Could you check a few things on this model? Use its own coordinates, in mm. Face numbers are marked on the shaded views. A direction names the side the tool comes from. Give positions to 0.01 mm unless a question says otherwise; leave off trailing zeros. Order: outer loops, then holes, each group sorted by start corner. A loop starts at its lowest first (then second) coordinate and runs counter-clockwise, first axis right, second up. Notation, with made-up numbers: (51.5, -27) -> (107.5, -27) arc R28 ccw to (107.5, 1) -> close; hole circle Ø11 at (52, 26.5). An arc over 180 degrees is marked (long way). Write each question's results on one line, items separated by ' | '.
Autodesk Inventor part; units mm, degrees
ref_plane "YZ Plane" through (0, 0, 0) normal (1, 0, 0) x (0, 1, 0)
ref_plane "XZ Plane" through (0, 0, 0) normal (0, 1, 0) x (-1, 0, 0)
ref_plane "XY Plane" through (0, 0, 0) normal (0, 0, 1) x (1, 0, 0)
sketch "Sketch1" plane through (0, 0, 0) normal (0, 0, 1) x (1, 0, 0)
  line L0 (-19.05, 38.1) -> (0, 38.1)
  line L1 (-19.05, -38.1) -> (-19.05, 38.1)
  line L2 (-38.1, -50.8) -> (-38.1, -38.1)
  line L3 (-19.05, -38.1) -> (-38.1, -38.1)
  line L4 (-38.1, -50.8) -> (0, -50.8)
  line L5 (0, 38.1) -> (0, -50.8)
  line L6 (0, -68.58) -> (0, 55.88)
  point P0 (0, 0)
revolve "Revolution1" add sketch "Sketch1" angle 360 about axis through (0, -10, 0) along (0, 1, 0)
sketch "Sketch2" plane through (0, -50.8, 0) normal (0, -1, 0) x (1, 0, 0)
  line L0 (25.4, 25.4) -> (-25.4, 25.4)
  line L1 (-25.4, 25.4) -> (-25.4, -25.4)
  line L2 (-25.4, -25.4) -> (25.4, -25.4)
  line L3 (25.4, -25.4) -> (25.4, 25.4)
  line L4 (25.4, 25.4) -> (-25.4, -25.4) construction
  line L5 (-25.4, 25.4) -> (25.4, -25.4) construction
  line L6 (25.4, 12.7) -> (-25.4, 12.7)
  line L7 (-25.4, 12.7) -> (-25.4, -12.7)
  line L8 (-25.4, -12.7) -> (25.4, -12.7)
  line L9 (25.4, -12.7) -> (25.4, 12.7)
  point P0 (0, 0)
  dimension "d5" = 50.8
  dimension "d6" = 50.8
extrude "Extrusion3" add sketch "Sketch2" along normal blind 50.8 contours L3 L8 L1 L6
fillet "Fillet2" radius 25.4 2 edges at (25.4, -101.6, 0) (-25.4, -101.6, 0)
sketch "Sketch4" plane through (-25.4, -50.8, 12.7) normal (0, 0, 1) x (1, 0, 0)
  arc A0 (0, -25.4) -> (50.8, -25.4) centre (25.4, -25.4) ccw
  line L0 (50.8, 0) -> (50.8, -25.4)
  line L1 (0, 0) -> (50.8, 0)
  line L2 (0, 0) -> (0, -25.4)
  circle A1 centre (25.4, -25.4) radius 9.525
  point P0 (25.4, 50.8)
  dimension "d16" = 19.05
extrude "Extrusion4" cut sketch "Sketch4" against normal blind 50.8 contours A1
properties part number "shock absorber bottom"
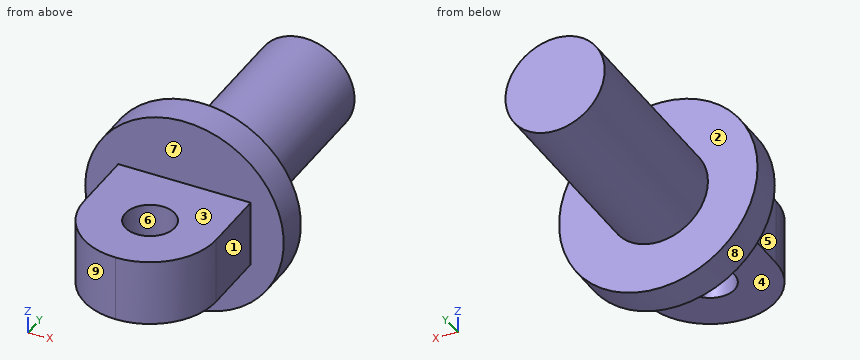
Q1. Suppose I cut it at D-D on x = -16. Please give me the cut outline in (y, z), and give its area (3 significant figures).
Here are the results:
outline: (-95.93, -12.7) -> (-50.8, -12.7) -> (-50.8, -34.58) -> (-38.1, -34.58) -> (-38.1, -10.34) -> (38.1, -10.34) -> (38.1, 10.34) -> (-38.1, 10.34) -> (-38.1, 34.58) -> (-50.8, 34.58) -> (-50.8, 12.7) -> (-95.93, 12.7) -> close | area: 3,600 mm²
Q2. Suppose I cut it at C-C on y = 3.5. Please give me the cut outline in (x, z).
Here are the results:
outline: circle Ø38.1 at (0, 0)
Q3. For the marked faces 1, 2, 3, 4 and 5, which set-ups out of +Z, -Z, +X, -X, +Y, -Y let a thin tool reach every point of the face, with its end or its side?
Here are the results:
face 1: +Z, -Z, +X, -Y | face 2: +Y | face 3: +Z, +X, -X, -Y | face 4: -Z, +X, -X, -Y | face 5: +Z, -Z, -X, -Y
Q4. Suppose I cut it at B-B on y = -80. Please give me the cut outline in (x, z).
Here are the results:
outline: (-25.11, -12.7) -> (-8.73, -12.7) -> (-8.73, 12.7) -> (-25.11, 12.7) -> close; (8.73, -12.7) -> (25.11, -12.7) -> (25.11, 12.7) -> (8.73, 12.7) -> close
Q5. Thinking about a two-plate mould opening in X: for the marked faces 6, 7, 8 and 9, which applies, +X half, -X half, draft (parallel to the pull), parting line (faces both ways), or undercut?
Here are the results:
face 6: undercut | face 7: draft | face 8: parting line | face 9: -X half
Q6. I need wall thicknesses on line 1 along Y through (x, z) = (0, -6.5) (3 decimals); line 2 along Z through (x, y) = (17, -85.5); line 3 along X through (y, z) = (-76, 4). Which ranges of each line are inside material? Lowest first, please.
Here are the results:
line 1: y = -101.6 to -85.725, -66.675 to 38.1 | line 2: z = -12.7 to 12.7 | line 3: x = -25.4 to -9.52, 9.52 to 25.4
Q7. I'm going to push flat-ended pins straight in: pin 1 Ø5 at (x, y) = (29.5, -83) entering from -Z; pin 2 Ø3 at (x, z) = (-27, 11) entering from +Y; pin 3 Ø12.5 at (y, z) = (-62, -4.5) entering from -X; pin 4 Ø12 at (x, y) = (-2, -0.5) entering from -Z. Where does each tip first touch, or does it pass through?
Here are the results:
pin 1: passes through | pin 2: stops at y = -38.1 | pin 3: stops at x = -25.4 | pin 4: stops at z = -19.05
